Source: CAD feature listing. Evaluate the final solid. Frame: model axes, mm. Face numbers are marked on the shaded views. A direction names the side the tool comes from. Give positions to 0.01 mm unless a question says otherwise; leave off trailing zeros. Order: outer loops, then holes, each group sorted by start corner. A loop starts at its lowest first (then second) coordinate and runs counter-clockwise, first axis right, second up.
1) First-contact query: P1, Ø12, axis at x = -17, y = 16.5, coming from the +Z side; P2, Ø10, axis at x = 1, z = 22.5, coming from the -Y side; P3, Ø3, axis at x = 28, y = 29, coming from the +Z side. Flat tips, straight axial feed; report the tip coordinate or a pass-through.
2) Section C-C, the plane x = 22. Return loops of the section in (y, z).
3) Section A-A, the plane x = 0. Return loops of the section in (y, z).
4) Section D-D, the plane y = 37. Return loops of the section in (x, z), plus the area to 3 significant figures.
5) Access query for the marked faces 1 and 2. Directions: +Z, -Z, +X, -X, +Y, -Y. A direction counts if a zero-diameter tool reaches every point of the face in a straight line with its end or side. Return the directions, or none.
6) Material intervals for line 1 (Z direction, x = -26, y = -37.5); line 2 (X direction, y = 48.5, z = 52); line 3 (X direction, y = 63, z = 23.5), sorted ascending.
7) Draft query along Z for the marked faces 3, 4 and 5. Return one class per face: released by +Z, released by -Z, zero draft, split by the parting line, or undercut.
8) Section B-B, the plane z = 30.5. Return loops of the section in (x, y), plus the area to 3 significant figures.
```python
from build123d import *

# Parameters (mm, degrees)
SKETCH1_W           = 72
SKETCH1_H           = 125
BOSS_EXTRUDE1_DEPTH = 5
SKETCH2_R           = 1.5
CUT_EXTRUDE6_DEPTH  = 5
BOSS_EXTRUDE2_DEPTH = 60
BOSS_EXTRUDE3_DEPTH = 119.5
SKETCH5_W           = 1
SKETCH5_H           = 65
SKETCH5_W_2         = 4
CUT_EXTRUDE7_DEPTH  = 158


with BuildPart() as part:
    # Sketch1 → Boss-Extrude1 (new body)
    with BuildSketch(Plane(origin=(0, 0, 0), x_dir=(-1, 0, 0), z_dir=(0, 0, 1))):
        with Locations((0, -8.5305)):
            Rectangle(SKETCH1_W, SKETCH1_H)
    extrude(amount=BOSS_EXTRUDE1_DEPTH)

    # Sketch2 → Cut-Extrude6 (cut)
    with BuildSketch(Plane(origin=(0, 0, 0), x_dir=(-1, 0, 0), z_dir=(0, 0, 1))):
        with Locations(Location((30.5, -67.5305, 0), (0, 0, 180))):
            Circle(SKETCH2_R)
        with Locations(Location((-30.5, -67.5305, 0), (0, 0, 180))):
            Circle(SKETCH2_R)
        with Locations(Location((30.5, 25.4695, 0), (0, 0, 180))):
            Circle(SKETCH2_R)
        with Locations(Location((-30.5, 25.4695, 0), (0, 0, 180))):
            Circle(SKETCH2_R)
        with Locations(Location((0, -21.0305, 0), (0, 0, 180))):
            Circle(SKETCH2_R)
    extrude(amount=CUT_EXTRUDE6_DEPTH, mode=Mode.SUBTRACT)

    # Sketch3 → Boss-Extrude2 (add)
    with BuildSketch(Plane.XY.offset(5)):
        Polygon((-30.5, -53.9695), (-30.5, 65.5305), (30.5, 65.5305), (30.5, -53.9695), (36, -53.9695), (36, 71.0305), (-36, 71.0305), (-36, -53.9695), align=None)
    extrude(amount=BOSS_EXTRUDE2_DEPTH)

    # Sketch4 → Boss-Extrude3 (add)
    with BuildSketch(Plane.XZ.offset(53.9695)):
        Polygon((-24, 18.356334593), (-29, 18.356334593), (-29, 49.356334593), (-24, 49.356334593), (-24, 54.356334593), (-30.5, 54.356334593), (-30.5, 13.356334593), (-24, 13.356334593), align=None)
        Polygon((29, 18.356334593), (24, 18.356334593), (24, 13.356334593), (30.5, 13.356334593), (30.5, 54.356334593), (24, 54.356334593), (24, 49.356334593), (29, 49.356334593), align=None)
    extrude(amount=-BOSS_EXTRUDE3_DEPTH)

    # Sketch5 → Cut-Extrude7 (cut)
    with BuildSketch(Plane(origin=(0, 71.0305, 0), x_dir=(1, 0, 0), z_dir=(0, 1, 0))):
        with Locations((-35.5, -32.5)):
            Rectangle(SKETCH5_W, SKETCH5_H)
        with Locations((-38, -32.5)):
            Rectangle(SKETCH5_W_2, SKETCH5_H)
        with Locations((38, -32.5)):
            Rectangle(SKETCH5_W_2, SKETCH5_H)
        with Locations((35.5, -32.5)):
            Rectangle(SKETCH5_W, SKETCH5_H)
    extrude(amount=-CUT_EXTRUDE7_DEPTH, mode=Mode.SUBTRACT)


solid = part.part
```
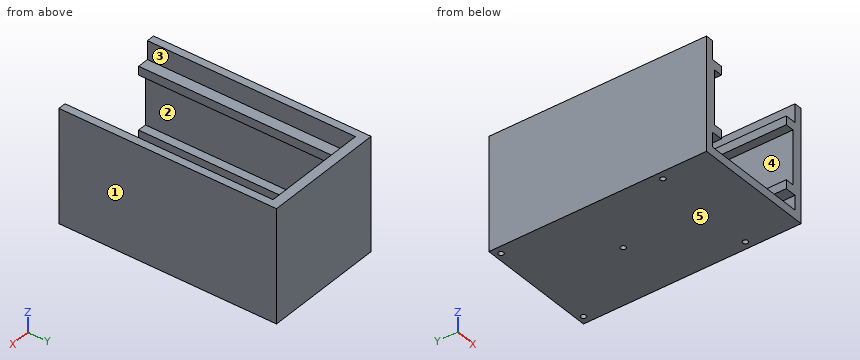
From the geometry:
1. P1: stops at z = 5
1. P2: stops at y = 65.53
1. P3: stops at z = 54.36
2. outline: (-53.97, 0) - (71.03, 0) - (71.03, 65) - (65.53, 65) - (65.53, 5) - (-53.97, 5) - close
3. outline: (-53.97, 0) - (19.53, 0) - (19.53, 5) - (-53.97, 5) - close; (22.53, 0) - (71.03, 0) - (71.03, 65) - (65.53, 65) - (65.53, 5) - (22.53, 5) - close
4. outline: (-35, 0) - (35, 0) - (35, 65) - (30.5, 65) - (30.5, 54.36) - (24, 54.36) - (24, 49.36) - (29, 49.36) - (29, 18.36) - (24, 18.36) - (24, 13.36) - (30.5, 13.36) - (30.5, 5) - (-30.5, 5) - (-30.5, 13.36) - (-24, 13.36) - (-24, 18.36) - (-29, 18.36) - (-29, 49.36) - (-24, 49.36) - (-24, 54.36) - (-30.5, 54.36) - (-30.5, 65) - (-35, 65) - close
4. area: 1,110 mm2
5. face 1: +Z, -Z, +X, +Y, -Y
5. face 2: -Y
6. line 1: z = 0 to 5, 13.36 to 18.36, 49.36 to 54.36
6. line 2: x = -35 to -24, 24 to 35
6. line 3: x = -35 to -29, 29 to 35
7. face 3: zero draft
7. face 4: undercut
7. face 5: released by -Z
8. outline: (-35, -53.97) - (-29, -53.97) - (-29, 65.53) - (29, 65.53) - (29, -53.97) - (35, -53.97) - (35, 71.03) - (-35, 71.03) - close
8. area: 1,820 mm2
